Input: part model. Units: mm. Frame: model coordinates. A direction names the side the tool comes from. Coordinates: 2 decimals unless noted, no trailing zeros. Loops run counter-clockwise (first coordinate to the right, second up) from the corner with the lowest first, then second, coordinate; pieces in that order, holes last. Notation, with made-up numbers: M -6,48.5 L 32,48.5 A30 cw 32,79.5 Z; hole C 89,-26 d11. An arc over 180 degrees is marked long. Use a Markdown table: item, result. Add a question column.
1. Section A-A on z = 7. Output: boundary loops of the cut face in (x, y).
2. Draft query along Z for faces 5 (the flat face through (7.49, -0.34, 17.64)), 6 (the flat face through (3, 0, 31.3)), 7 (the cylindrical face through (2.9, 0, -1)). Return one class per face: +Z half, -Z half, draft (parallel to the pull), parting line (faces both ways), or undercut.
3. Pin query (flat end, axial travel): pin 1 (4 mm diameter, centred on y = -2, z = 3, fed in from +X); pin 2 (2 mm diameter, centred on x = -4.5, z = 25, fed in from +Y); pin 3 (1.5 mm diameter, centred on x = 1.5, z = 5, fed in from +Y); pin 4 (2.5 mm diameter, centred on x = -2, y = -2.5, fed in from +Z). Return the tip coordinate at first contact, or that it passes through.
4. Line query: L1, parallel to Y at x = 0, z = 31.45; L2, parallel to Z at x = 1, y = 4.25; L3, parallel to X at y = 0.75, z = 16. Output: solid intervals per line, ascending. Write a range as [from, to].
5. Section B-B on z = 17. Output: boundary loops of the cut face in (x, y), then the cut area to 3 significant figures.
6. Set-up query: faces 1 (the flat face through (3.5, 0, -2)), 2 (the flat face through (7.49, -0.34, 25.14)), 3 (the flat face through (-1, -3, 31.3)), 4 (the cylindrical face through (-4.1, 0, -1)). Return all of +Z, -Z, +X, -X, +Y, -Y with unobstructed straight access to the full face (end or side cutting, diameter ignored); none if empty.
```python
from build123d import *

# Parameters (mm, degrees)
SKETCH_1_R          = 8
EXTRUDE_1_DEPTH     = 31.5
SKETCH_2_R          = 5.5
CUT_EXTRUDE_1_DEPTH = 0.2
CUT_EXTRUDE_2_DEPTH = 0.2
FILLET_1_R          = 0.25
SKETCH_5_R          = 0.6
EXTRUDE_2_DEPTH     = 2
WRAP_START          = 8.527777778
WRAP_2_DEPTH        = 3.263888889
WRAP_START_2        = 16.027777778
WRAP_2_2_DEPTH      = 3.263888889
WRAP_START_3        = 23.527777778
WRAP_2_3_DEPTH      = 3.263888889


# Read off the part's stored shape, not the designer's step: 包覆2
with BuildPart() as part:
    # 草图1 → 凸台-拉伸1 (new body)
    with BuildSketch(Plane.XY):
        Circle(SKETCH_1_R)
    extrude(amount=EXTRUDE_1_DEPTH)

    # 草图2 → 切除-拉伸1 (cut)
    with BuildSketch(Plane.XY.offset(31.5)):
        Circle(SKETCH_2_R)
    extrude(amount=-CUT_EXTRUDE_1_DEPTH, mode=Mode.SUBTRACT)

    # 草图3 → 切除-拉伸2 (cut)
    with BuildSketch(Plane.XY.offset(31.3)):
        with BuildLine():
            Line((-0.04330127, 0.025), (-0.028867513, 0.05))
            Line((-0.028867513, 0.05), (-5.499772723, 0.05))
            ThreePointArc((-5.499772723, 0.05), (-5.5, 0), (-5.499772723, -0.05))
            Line((-5.499772723, -0.05), (-0.028867513, -0.05))
            Line((-0.028867513, -0.05), (-0.04330127, -0.025))
            Line((-0.04330127, -0.025), (0, 0))
            Line((0, 0), (-0.04330127, 0.025))
        make_face()
        with BuildLine():
            Line((0.04330127, -0.025), (0, 0))
            Line((0, 0), (0, -0.05))
            Line((0, -0.05), (-0.028867513, -0.05))
            Line((-0.028867513, -0.05), (2.706585091, -4.787942893))
            ThreePointArc((2.706585091, -4.787942893), (2.75, -4.763139721), (2.793187631, -4.737942893))
            Line((2.793187631, -4.737942893), (0.057735027, 0))
            Line((0.057735027, 0), (0.04330127, -0.025))
        make_face()
        with BuildLine():
            Line((-0.028867513, 0.05), (0, 0.05))
            Line((0, 0.05), (0, 0))
            Line((0, 0), (0.04330127, 0.025))
            Line((0.04330127, 0.025), (0.057735027, 0))
            Line((0.057735027, 0), (2.793187631, 4.737942893))
            ThreePointArc((2.793187631, 4.737942893), (2.75, 4.763139721), (2.706585091, 4.787942893))
            Line((2.706585091, 4.787942893), (-0.028867513, 0.05))
        make_face()
        Polygon((0, 0), (0, 0.05), (-0.028867513, 0.05), (-0.04330127, 0.025), align=None)
        Polygon((0, -0.05), (0, 0), (-0.04330127, -0.025), (-0.028867513, -0.05), align=None)
        Polygon((0.04330127, 0.025), (0, 0), (0.04330127, -0.025), (0.057735027, 0), align=None)
    extrude(amount=-CUT_EXTRUDE_2_DEPTH, mode=Mode.SUBTRACT)

    # 草图4 → 切除-旋转1 (revolve, cut)
    with BuildSketch(Plane(origin=(0, 0, 0), x_dir=(1, 0, 0), z_dir=(0, 1, 0))):
        with BuildLine():
            Line((-8.318421305, -2.223982894), (-8.318421305, -6.342581877))
            ThreePointArc((-8.318421305, -6.342581877), (-7.5, -4.283282386), (-8.318421305, -2.223982894))
        make_face()
    revolve(axis=Axis((0, 0, 0), (0, 0, 1)), mode=Mode.SUBTRACT)

    # 圆角1
    fillet_1_edges = [part.edges().sort_by_distance(p)[0] for p in [
        (0, 8, 5.941594781),
        (0, -8, 2.62496999),
    ]]
    fillet(fillet_1_edges, radius=FILLET_1_R)

    # 草图5 → 凸台-拉伸2 (add)
    with BuildSketch(Plane(origin=(0, 0, 0), x_dir=(-1, 0, 0), z_dir=(0, 0, -1))):
        with Locations(Location((3.5, 0, 0), (0, 0, 180))):
            Circle(SKETCH_5_R)
        with Locations(Location((-3.5, 0, 0), (0, 0, 180))):
            Circle(SKETCH_5_R)
    extrude(amount=EXTRUDE_2_DEPTH)

    # 包覆2 outline → 包覆2 (cut)
    with BuildSketch(Plane.XY.offset(WRAP_START)):
        with BuildLine():
            Line((7.998541229, -0.152768492), (6.998723575, -0.13367243))
            ThreePointArc((6.998723575, -0.13367243), (6.996389817, -0.224787737), (6.992869893, -0.315864933))
            Line((6.992869893, -0.315864933), (7.991851307, -0.360988495))
            ThreePointArc((7.991851307, -0.360988495), (7.995874077, -0.256900271), (7.998541229, -0.152768492))
        make_face()
    extrude(amount=WRAP_2_DEPTH, mode=Mode.SUBTRACT)

    # Wrap 2 2 outline → Wrap 2 2 (cut)
    with BuildSketch(Plane.XY.offset(WRAP_START_2)):
        with BuildLine():
            Line((7.998541229, -0.152768492), (6.998723575, -0.13367243))
            ThreePointArc((6.998723575, -0.13367243), (6.996389817, -0.224787737), (6.992869893, -0.315864933))
            Line((6.992869893, -0.315864933), (7.991851307, -0.360988495))
            ThreePointArc((7.991851307, -0.360988495), (7.995874077, -0.256900271), (7.998541229, -0.152768492))
        make_face()
    extrude(amount=WRAP_2_2_DEPTH, mode=Mode.SUBTRACT)

    # Wrap 2 3 outline → Wrap 2 3 (cut)
    with BuildSketch(Plane.XY.offset(WRAP_START_3)):
        with BuildLine():
            Line((7.998541229, -0.152768492), (6.998723575, -0.13367243))
            ThreePointArc((6.998723575, -0.13367243), (6.996389817, -0.224787737), (6.992869893, -0.315864933))
            Line((6.992869893, -0.315864933), (7.991851307, -0.360988495))
            ThreePointArc((7.991851307, -0.360988495), (7.995874077, -0.256900271), (7.998541229, -0.152768492))
        make_face()
    extrude(amount=WRAP_2_3_DEPTH, mode=Mode.SUBTRACT)


solid = part.part
```
Answers below:
| question | item | result |
|---|---|---|
| 1 | outline | C 0,0 d16 |
| 2 | face 5 | undercut |
| 2 | face 6 | +Z half |
| 2 | face 7 | draft |
| 3 | pin 1 | stops at x = 8 |
| 3 | pin 2 | stops at y = 7.19 |
| 3 | pin 3 | stops at y = 7.76 |
| 3 | pin 4 | stops at z = 31.3 |
| 4 | L1 | y = [-8, -5.5], [5.5, 8] |
| 4 | L2 | z = [0, 31.3] |
| 4 | L3 | x = [-7.96, 7.96] |
| 5 | outline | M 6.99,-0.32 A7 ccw 7,-0.13 L 8,-0.15 A8 ccw long 7.99,-0.36 Z |
| 5 | area | 201 mm² |
| 6 | face 1 | -Z, +X, -X, +Y, -Y |
| 6 | face 2 | +X |
| 6 | face 3 | +Z |
| 6 | face 4 | -Z |
